Source: CAD feature listing. Evaluate the final solid. Frame: model axes, mm. Round coordinates to 2 decimals unless told otherwise and drop trailing zeros. Write each loop counter-clockwise with the first axis right and the second up, starting at its lowest first coordinate (ties: lowest second). Pieces come first, ordered by that corner, then holes.
Autodesk Fusion 360 part; units mm, degrees
sketch "Boceto1" plane through (0, 0, 0) normal (1, 0, 0) x (0, 1, 0)
  line L0 (0, 0) -> (90, 0)
  line L1 (90, 5) -> (0, 5)
  line L2 (0, 5) -> (-0.8775, 5)
  line L3 (90, 5) -> (90.8775, 5)
  line L4 (0, 0) -> (-2, 0)
  line L5 (90, 0) -> (91.5, 0)
  circle A0 centre (94, 2.5) radius 1.5
  circle A1 centre (-4, 2.5) radius 1.5
  arc A2 (-0.8775, 5) -> (-0.8775, 0) centre (-4, 2.5) ccw
  arc A3 (90.8775, 0) -> (90.8775, 5) centre (94, 2.5) ccw
  dimension "d1" = 90
  dimension "d2" = 5
  dimension "d4" = 3
  dimension "d5" = 3
extrude "Extruir1" add sketch "Boceto1" along normal blind 1.5
sketch "Boceto2" plane through (1.5, 0, 0) normal (1, 0, 0) x (0, 1, 0)
  circle A0 centre (94, 2.5) radius 1.5
  circle A1 centre (-4, 2.5) radius 1.5
  line L0 (-0.8775, 0) -> (90.8775, 0)
  arc A2 (90.8775, 0) -> (90.8775, 5) centre (94, 2.5) ccw
  line L1 (90.8775, 5) -> (-0.8775, 5)
  arc A3 (-0.8775, 5) -> (-0.8775, 0) centre (-4, 2.5) ccw
1) Pull-direction query (Y, two-part tool) for faces 1 (the face through (0.7, 98, 2.6)), 2 (the face through (1.5, 44, 3)); classes: released by +Y, released by -Y, zero draft, split by the parting line, or undercut.
Taken from the geometry:
face 1: undercut
face 2: zero draft
2) Section query C-C on x = 0.5. Return the cut outline in (y, z), then the cut area to 3 significant figures.
Taken from the geometry:
outline: (-0.88, 0) - (90.88, 0) arc R4 ccw (long way) to (90.88, 5) - (-0.88, 5) arc R4 ccw (long way) to start; hole circle Ø3 at (-4, 2.5); hole circle Ø3 at (94, 2.5)
area: 539 mm2
3) Material intervals for line 1 (Y direction, x = 1.3, z = 2.75); line 2 (Z direction, x = 1, y = 94); line 3 (Y direction, x = 1.2, z = 2), sorted ascending.
Taken from the geometry:
line 1: y = -7.99 to -5.48, -2.52 to 92.52, 95.48 to 97.99
line 2: z = -1.5 to 1, 4 to 6.5
line 3: y = -7.97 to -5.41, -2.59 to 92.59, 95.41 to 97.97
4) Section query A-A on y = -4. Return the cut outline in (x, z), then the cut area to 3 significant figures.
Taken from the geometry:
outline: (0, -1.5) - (1.5, -1.5) - (1.5, 1) - (0, 1) - close; (0, 4) - (1.5, 4) - (1.5, 6.5) - (0, 6.5) - close
area: 7.50 mm2
5) Section query B-B on z = 2.5. Return the cut outline in (x, y).
Taken from the geometry:
outline: (0, -8) - (1.5, -8) - (1.5, -5.5) - (0, -5.5) - close; (0, -2.5) - (1.5, -2.5) - (1.5, 92.5) - (0, 92.5) - close; (0, 95.5) - (1.5, 95.5) - (1.5, 98) - (0, 98) - close
6) Contact query for a flat-ended pin moving along its axis: P1, Ø4, axis at y = 53.5, z = 5.5, coming from the +X side. Output: stop coordinate, or through.
Taken from the geometry:
P1: stops at x = 1.5
7) Section query D-D on y = 41. Return the cut outline in (x, z).
Taken from the geometry:
outline: (0, 0) - (1.5, 0) - (1.5, 5) - (0, 5) - close
